Autodesk Inventor part; units mm, degrees
ref_plane "YZ Plane" through (0, 0, 0) normal (1, 0, 0) x (0, 1, 0)
ref_plane "XZ Plane" through (0, 0, 0) normal (0, 1, 0) x (-1, 0, 0)
ref_plane "XY Plane" through (0, 0, 0) normal (0, 0, 1) x (1, 0, 0)
sketch "Sketch1" plane through (0, 0, 0) normal (0, 0, 1) x (1, 0, 0)
  circle A0 centre (0, 0) radius 3
  dimension "d0" = 6
extrude "Extrusion1" add sketch "Sketch1" along normal mid plane 46
sketch "Sketch2" plane through (0, 0, 23) normal (0, 0, 1) x (1, 0, 0)
  point P0 (0, 0)
  point P1 (0, 0)
hole "Hole1" at (0, 0, 23) direction (0, 0, -1) diameter 2.459 depth 8.8 tip angle 118
sketch "Sketch3" plane through (0, 0, 0) normal (0, 1, 0) x (-1, 0, 0)
  line L0 (3, -23) -> (3, 23)
  line L1 (3, 18) -> (2.5, 18)
  line L2 (2.5, 18) -> (2.5, 13)
  line L3 (2.5, 13) -> (3, 13)
  line L4 (3, 13) -> (3, 18)
  line L5 (-3, 18) -> (-2.5, 18)
  line L6 (-2.5, 18) -> (-2.5, 13)
  line L7 (-2.5, 13) -> (-3, 13)
  line L8 (-3, 13) -> (-3, 18)
  line L9 (3, 23) -> (-3, 23)
  point P0 (0, 0)
  dimension "d10" = 0.5
  dimension "d11" = 5
  dimension "d12" = 0.5
  dimension "d16" = 5
  dimension "d19" = 5
  dimension "d20" = 6
  dimension "d21" = 6
extrude "Extrusion2" cut sketch "Sketch3" along normal through all both and the other way through all
mirror "Mirror1" about plane through (0, 0, 0) normal (0, 0, 1) of "Hole1"
equation "\"d10\" = d12"
equation "\"d20\" = d21"
properties part number "Top_Separator Weight 2" material "Aluminum 6061"
Geometry check sheet. Reference: the model listing, model coordinates, mm. A direction names the side the tool comes from. Coordinates: 2 decimals unless noted, no trailing zeros. Order: outer loops, then holes, each group sorted by start corner. A loop starts at its lowest first (then second) coordinate and runs counter-clockwise, first axis right, second up.
Item 1: Section check C-C (y = 2.3). Enter the section's corners in (x, z).
Item 2: Tool access check on faces 5 (the flat face through (1, -1, 23)), 6 (the flat face through (-2.5, 0, 16)), 7 (the cylindrical face through (-0.748, 0.976, -18.538)). Record the directions out of +Z, -Z, +X, -X, +Y, -Y that give a thin tool (end or side, any length) a straight path to the whole face; none if there is none.
Item 3: Scan lines: line 1 along X through (y, z) = (0, -16.5); line 2 along Y through (x, z) = (-0.8, -15.5). Record each from-to range of solid material in increasing order.
Item 4: Section check A-A (z = -17). Enter the section's corners in (x, y).
Item 5: Section check D-D (x = -2.05). Enter the section's corners in (y, z), plus the area to 3 significant figures.
Item 6: Section check B-B (z = -10). Enter the section's corners in (x, y), plus the area to 3 significant figures.
Item 7: Depth check by flat-ended pin: pin 1 (0.6 mm diameter, centred on x = 3, y = 1, fed in from +Z); pin 2 (3.5 mm diameter, centred on y = 0, z = 16, fed in from -X); pin 3 (1 mm diameter, centred on y = 0.5, z = 15.5, fed in from +X). Enter the tip coordinate at first touch or a pass-through.
Item 8: Mould release check, pull along X, two halves, no side actions. Record for faces 1 (the cylindrical face through (-3, 0, 0)), 2 (the cylindrical face through (0.748, 0.976, 18.538)), 3 (the conical face through (0.21, 0.03, 13.59)), 4 (the flat face through (2.5, 0, 16)): released by +X, released by -X, zero draft, split by the parting line, or undercut.
Check sheet entries:
1. outline: (-1.93, -23) - (1.93, -23) - (1.93, 23) - (-1.93, 23) - close
2. face 5: +Z, +X, -X, +Y, -Y
2. face 6: -X, +Y, -Y
2. face 7: -Z
3. line 1: x = -3 to -1.23, 1.23 to 3
3. line 2: y = -2.89 to -0.93, 0.93 to 2.89
4. outline: circle Ø6 at (0, 0); hole circle Ø2.46 at (0, 0)
5. outline: (-2.19, -23) - (2.19, -23) - (2.19, 23) - (-2.19, 23) - close
5. area: 202 mm2
6. outline: circle Ø6 at (0, 0)
6. area: 28.3 mm2
7. pin 1: stops at z = 23
7. pin 2: stops at x = -2.5
7. pin 3: stops at x = 2.5
8. face 1: split by the parting line
8. face 2: undercut
8. face 3: undercut
8. face 4: released by +X
